Check sheet for the modelled part. Datum: model origin and axes. Units: mm. A direction names the side the tool comes from. Round coordinates to 2 decimals unless told otherwise and drop trailing zeros. Order: outer loops, then holes, each group sorted by start corner. A loop starts at its lowest first (then second) coordinate and runs counter-clockwise, first axis right, second up.
Autodesk Inventor part; units mm, degrees
ref_plane "YZ Plane" through (0, 0, 0) normal (1, 0, 0) x (0, 1, 0)
ref_plane "XZ Plane" through (0, 0, 0) normal (0, 1, 0) x (-1, 0, 0)
ref_plane "XY Plane" through (0, 0, 0) normal (0, 0, 1) x (1, 0, 0)
sketch "Boceto1" plane through (0, 0, 0) normal (0, 1, 0) x (-1, 0, 0)
  circle A0 centre (0, 0) radius 50
  dimension "d0" = 100
extrude "Extrusión1" add sketch "Boceto1" along normal blind 5
sketch "Boceto2" plane through (0, 5, 0) normal (0, 1, 0) x (1, 0, 0)
  circle A0 centre (0, 0) radius 37.5 construction
  line L0 (-37.5, 0) -> (-18.75, 32.476) construction
  line L1 (-18.75, 32.476) -> (18.75, 32.476) construction
  line L2 (18.75, 32.476) -> (37.5, 0) construction
  line L3 (37.5, 0) -> (18.75, -32.476) construction
  line L4 (18.75, -32.476) -> (-18.75, -32.476) construction
  line L5 (-18.75, -32.476) -> (-37.5, 0) construction
  circle A1 centre (-18.75, -32.476) radius 3.5
  circle A2 centre (-37.5, 0) radius 3.5
  circle A3 centre (-18.75, 32.476) radius 3.5
  circle A4 centre (18.75, 32.476) radius 3.5
  circle A5 centre (37.5, 0) radius 3.5
  circle A6 centre (18.75, -32.476) radius 3.5
  dimension "d3" = 75
  dimension "d4" = 7
  dimension "d5" = 7
  dimension "d6" = 7
  dimension "d7" = 7
  dimension "d8" = 7
  dimension "d9" = 7
extrude "Extrusión2" cut sketch "Boceto2" against normal blind 2
sketch "Boceto3" plane through (0, 5, 0) normal (0, 1, 0) x (1, 0, 0)
  circle A0 centre (0, 0) radius 37.5 construction
  circle A1 centre (37.5, 0) radius 3.5
  line L0 (37.5, 0) -> (18.75, -32.476) construction
  line L1 (18.75, -32.476) -> (-18.75, -32.476) construction
  line L2 (-18.75, -32.476) -> (-37.5, 0) construction
  line L3 (-37.5, 0) -> (-18.75, 32.476) construction
  line L4 (-18.75, 32.476) -> (18.75, 32.476) construction
  line L5 (18.75, 32.476) -> (37.5, 0) construction
  circle A2 centre (-37.5, 0) radius 1.75
  circle A3 centre (-18.75, -32.476) radius 1.75
  circle A4 centre (18.75, -32.476) radius 1.75
  circle A5 centre (37.5, 0) radius 1.75
  circle A6 centre (18.75, 32.476) radius 1.75
  circle A7 centre (-18.75, 32.476) radius 1.75
  dimension "d12" = 75
  dimension "d13" = 3.5
  dimension "d14" = 3.5
  dimension "d15" = 3.5
  dimension "d16" = 3.5
  dimension "d17" = 3.5
  dimension "d18" = 3.5
extrude "Extrusión3" cut sketch "Boceto3" along normal mid plane 10 contours A2 | A3 | A4 | A5 | A6 | A7
Item 1: Sectioned sample at B-B (y = 1.45). Record the cut outline in (x, z), and give its area (3 significant figures).
Answer:
outline: circle Ø100 at (0, 0); hole circle Ø3.5 at (-37.5, 0); hole circle Ø3.5 at (-18.75, -32.48); hole circle Ø3.5 at (-18.75, 32.48); hole circle Ø3.5 at (18.75, -32.48); hole circle Ø3.5 at (18.75, 32.48); hole circle Ø3.5 at (37.5, 0)
area: 7,800 mm2
Item 2: Release check for a two-part mould opening along Z. For faces 3 (the flat face through (1, 5, 1)), 4 (the cylindrical face through (-47.69, 2.46, -15.02)), 5 (the cylindrical face through (39.117, 1.521, 0.67)) record: released by +Z, released by -Z, zero draft, split by the parting line, or undercut.
Answer:
face 3: zero draft
face 4: split by the parting line
face 5: undercut
Item 3: Sectioned sample at C-C (x = -37.5). Record the cut outline in (y, z).
Answer:
outline: (0, -33.07) - (5, -33.07) - (5, -3.5) - (3, -3.5) - (3, -1.75) - (0, -1.75) - close; (0, 1.75) - (3, 1.75) - (3, 3.5) - (5, 3.5) - (5, 33.07) - (0, 33.07) - close
Item 4: Scan lines: line 1 along Z through (x, y) = (-18, 4.85); line 2 along X through (y, z) = (3.25, 1); line 3 along Z through (x, y) = (18.75, 4.1). Record each from-to range of solid material in increasing order.
Answer:
line 1: z = -46.65 to -35.89, -29.06 to 29.06, 35.89 to 46.65
line 2: x = -49.99 to -40.85, -34.15 to 34.15, 40.85 to 49.99
line 3: z = -46.35 to -35.98, -28.98 to 28.98, 35.98 to 46.35
Item 5: Sectioned sample at A-A (x = -18.75). Record the cut outline in (y, z), and give its area (3 significant figures).
Answer:
outline: (0, -46.35) - (5, -46.35) - (5, -35.98) - (3, -35.98) - (3, -34.23) - (0, -34.23) - close; (0, -30.73) - (3, -30.73) - (3, -28.98) - (5, -28.98) - (5, 28.98) - (3, 28.98) - (3, 30.73) - (0, 30.73) - close; (0, 34.23) - (3, 34.23) - (3, 35.98) - (5, 35.98) - (5, 46.35) - (0, 46.35) - close
area: 415 mm2
Item 6: Sectioned sample at D-D (z = 40.5). Record the cut outline in (x, y), and give its area (3 significant figures).
Answer:
outline: (-29.32, 0) - (29.32, 0) - (29.32, 5) - (-29.32, 5) - close
area: 293 mm2
Item 7: Access from +Z, -Z, +X, -X, +Y, -Y to the whole of each face (thin tool, end or side, straight path). Record for faces 1 (the cylindrical face through (-20.04, 1.521, 31.293)), 2 (the flat face through (20, 3, -31)).
Answer:
face 1: +Y, -Y
face 2: +Y
Item 8: Go/stop test with flat-tipped pins: P1, Ø3, axis at x = -34, y = 1.5, coming from the -Z side; P2, Ø3, axis at y = 1.5, z = -4, coming from the +X side; P3, Ø6.5, axis at x = -18.75, z = -32.476, coming from the +Y side; P4, Ø3, axis at x = 37.5, z = 0, coming from the -Y side. Record where each tip stops, or that it passes through.
Answer:
P1: stops at z = -38
P2: stops at x = 49.94
P3: stops at y = 3
P4: passes through
